from build123d import *

# Parameters (mm, degrees)
PAD_DEPTH     = 20.07
POCKET_DEPTH  = 18.42
SKETCH002_R   = 3
HOLE_DEPTH    = 25
SKETCH003_R   = 3
HOLE001_DEPTH = 25
SKETCH004_R   = 3
HOLE002_DEPTH = 25
SKETCH005_R   = 3
HOLE003_DEPTH = 25
SKETCH006_R   = 3
HOLE004_DEPTH = 25
SKETCH007_R   = 3
HOLE005_DEPTH = 25
SKETCH008_R   = 3
HOLE006_DEPTH = 25
FILLET_R      = 1.5
SKETCH009_R   = 3
HOLE007_DEPTH = 25
SKETCH010_R   = 3
HOLE008_DEPTH = 25
SKETCH011_R   = 3
HOLE009_DEPTH = 25
SKETCH012_R   = 3
HOLE010_DEPTH = 25
SKETCH013_R   = 3
HOLE011_DEPTH = 25
SKETCH014_R   = 3
HOLE012_DEPTH = 25
SKETCH015_R   = 3
HOLE013_DEPTH = 25


with BuildPart() as part:
    # Sketch → Pad (new body)
    with BuildSketch(Plane.XY):
        with BuildLine():
            Line((18.834122, 40.018788), (92.644122, 40.018788))
            ThreePointArc((95.644122, 37.018788), (94.765442, 39.140108), (92.644122, 40.018788))
            Line((95.644122, 37.018788), (95.644122, 5.428788))
            ThreePointArc((92.644122, 2.428788), (94.765442, 3.307467), (95.644122, 5.428788))
            Line((92.644122, 2.428788), (18.834122, 2.428788))
            ThreePointArc((15.834122, 5.428788), (16.712801, 3.307467), (18.834122, 2.428788))
            Line((15.834122, 5.428788), (15.834122, 37.018788))
            ThreePointArc((18.834122, 40.018788), (16.712801, 39.140108), (15.834122, 37.018788))
        make_face()
    extrude(amount=PAD_DEPTH)

    # Sketch001 (on Face9 of Pad) → Pocket (cut)
    with BuildSketch(Plane(origin=(0, 0, 0), x_dir=(1, 0, 0), z_dir=(0, 0, -1))):
        with BuildLine():
            Line((19.344122, -2.933788), (92.134122, -2.933788))
            ThreePointArc((95.134122, -5.933788), (94.255442, -3.812467), (92.134122, -2.933788))
            Line((95.134122, -5.933788), (95.134122, -36.513788))
            ThreePointArc((92.134122, -39.513788), (94.255442, -38.635108), (95.134122, -36.513788))
            Line((92.134122, -39.513788), (19.344122, -39.513788))
            ThreePointArc((16.344122, -36.513788), (17.222801, -38.635108), (19.344122, -39.513788))
            Line((16.344122, -36.513788), (16.344122, -5.933788))
            ThreePointArc((19.344122, -2.933788), (17.222801, -3.812467), (16.344122, -5.933788))
        make_face()
    extrude(amount=-POCKET_DEPTH, mode=Mode.SUBTRACT)

    # Sketch002 (on Face5 of Pocket) → Hole (cut)
    with BuildSketch(Plane.XY.offset(20.07)):
        with Locations((55.739122, 30.621288)):
            Circle(SKETCH002_R)
    extrude(amount=-HOLE_DEPTH, mode=Mode.SUBTRACT)

    # Sketch003 (on Face5 of Hole) → Hole001 (cut)
    with BuildSketch(Plane.XY.offset(20.07)):
        with Locations((45.501322, 30.621288)):
            Circle(SKETCH003_R)
    extrude(amount=-HOLE001_DEPTH, mode=Mode.SUBTRACT)

    # Sketch004 (on Face5 of Hole001) → Hole002 (cut)
    with BuildSketch(Plane.XY.offset(20.07)):
        with Locations((35.290522, 30.621288)):
            Circle(SKETCH004_R)
    extrude(amount=-HOLE002_DEPTH, mode=Mode.SUBTRACT)

    # Sketch005 (on Face5 of Hole002) → Hole003 (cut)
    with BuildSketch(Plane.XY.offset(20.07)):
        with Locations((25.079722, 30.621288)):
            Circle(SKETCH005_R)
    extrude(amount=-HOLE003_DEPTH, mode=Mode.SUBTRACT)

    # Sketch006 (on Face5 of Hole003) → Hole004 (cut)
    with BuildSketch(Plane.XY.offset(20.07)):
        with Locations((65.922922, 30.621288)):
            Circle(SKETCH006_R)
    extrude(amount=-HOLE004_DEPTH, mode=Mode.SUBTRACT)

    # Sketch007 (on Face5 of Hole004) → Hole005 (cut)
    with BuildSketch(Plane.XY.offset(20.07)):
        with Locations((76.133722, 30.621288)):
            Circle(SKETCH007_R)
    extrude(amount=-HOLE005_DEPTH, mode=Mode.SUBTRACT)

    # Sketch008 (on Face5 of Hole005) → Hole006 (cut)
    with BuildSketch(Plane.XY.offset(20.07)):
        with Locations((86.344522, 30.621288)):
            Circle(SKETCH008_R)
    extrude(amount=-HOLE006_DEPTH, mode=Mode.SUBTRACT)

    # Fillet
    fillet_edges = [part.edges().sort_by_distance(p)[0] for p in [
        (55.739122, 40.018788, 20.07),
    ]]
    fillet(fillet_edges, radius=FILLET_R)

    # Sketch009 (on Face8 of Fillet) → Hole007 (cut)
    with BuildSketch(Plane.XY.offset(20.07)):
        with Locations((55.739122, 11.826288)):
            Circle(SKETCH009_R)
    extrude(amount=-HOLE007_DEPTH, mode=Mode.SUBTRACT)

    # Sketch010 (on Face8 of Hole007) → Hole008 (cut)
    with BuildSketch(Plane.XY.offset(20.07)):
        with Locations((45.501322, 11.826288)):
            Circle(SKETCH010_R)
    extrude(amount=-HOLE008_DEPTH, mode=Mode.SUBTRACT)

    # Sketch011 (on Face8 of Hole008) → Hole009 (cut)
    with BuildSketch(Plane.XY.offset(20.07)):
        with Locations((35.290522, 11.826288)):
            Circle(SKETCH011_R)
    extrude(amount=-HOLE009_DEPTH, mode=Mode.SUBTRACT)

    # Sketch012 (on Face8 of Hole009) → Hole010 (cut)
    with BuildSketch(Plane.XY.offset(20.07)):
        with Locations((25.079722, 11.826288)):
            Circle(SKETCH012_R)
    extrude(amount=-HOLE010_DEPTH, mode=Mode.SUBTRACT)

    # Sketch013 (on Face8 of Hole010) → Hole011 (cut)
    with BuildSketch(Plane.XY.offset(20.07)):
        with Locations((65.922922, 11.826288)):
            Circle(SKETCH013_R)
    extrude(amount=-HOLE011_DEPTH, mode=Mode.SUBTRACT)

    # Sketch014 (on Face8 of Hole011) → Hole012 (cut)
    with BuildSketch(Plane.XY.offset(20.07)):
        with Locations((76.133722, 11.826288)):
            Circle(SKETCH014_R)
    extrude(amount=-HOLE012_DEPTH, mode=Mode.SUBTRACT)

    # Sketch015 (on Face8 of Hole012) → Hole013 (cut)
    with BuildSketch(Plane.XY.offset(20.07)):
        with Locations((86.344522, 11.826288)):
            Circle(SKETCH015_R)
    extrude(amount=-HOLE013_DEPTH, mode=Mode.SUBTRACT)


solid = part.part
Here's how the part is built. I have some questions about the finished solid (model axes, mm). A direction names the side the tool comes from. Give positions to 0.01 mm unless a question says otherwise; leave off trailing zeros. Order: outer loops, then holes, each group sorted by start corner. A loop starts at its lowest first (then second) coordinate and runs counter-clockwise, first axis right, second up. Notation, with made-up numbers: M -27.75,52.5 L 19.25,52.5 A25 cw 19.25,66.5 Z; hole C 32,-23.5 d1. An arc over 180 degrees is marked long. Answer as a JSON object with one key per item and string values. Group by question number.
1) We'd pull the mould along Y, two halves only. Please class faces 3 (the cylindrical face through (43.29, 32.65, 19.26)), 4 (the cylindrical face through (16.69, 3.33, 9.16)), 5 (the cylindrical face through (94.789, 39.117, 9.155)): pulls with the +Y half, pulls with the -Y half, needs draft (parallel to the pull), parting line crosses it, or undercut.
2) Suppose I cut it at C-C, the plane x = 52. Write out the boundary of the cut face in (y, z).
3) Suppose I cut it at A-A, the plane z = 12.5. Write out the boundary of the cut face in (x, y).
4) I'm going to push flat-ended pins straight in: pin 1 Ø5 at (x, y) = (35.29, 11.83) entering from -Z; pin 2 Ø7 at (x, y) = (25.08, 30.62) entering from -Z. Where does each tip first touch, or does it pass through?
5) Suppose I cut it at B-B, the plane y = 19.5. Write out the boundary of the cut face in (x, z).
6) Please list where these lines run through material, in increasing order: L1, parallel to Y at x = 89.5, z = 16.25; L2, parallel to X at y = 10, z = 5; L3, parallel to Z at x = 53, y = 16. Write a range as [from, to].
7) Suppose I cut it at D-D, the plane x = 78. Write out the boundary of the cut face in (y, z).
8) On a 3-axis mill with a long thin cutter (end or side, diameter ignored), from which of +Z, -Z, +X, -X, +Y, -Y can I reach the whole of each face in a straight line? I mean faces 1 (the flat face through (55, 2.934, 9)), 2 (the flat face through (95.644, 21, 9)). Say none if no direction works.
Results found:
{
 "1": {"face 3": "undercut", "face 4": "pulls with the -Y half", "face 5": "pulls with the +Y half"},
 "2": {"outline": "M 2.43,0 L 2.93,0 L 2.93,18.42 L 39.51,18.42 L 39.51,0 L 40.02,0 L 40.02,18.57 A1.5 ccw 38.52,20.07 L 3.93,20.07 A1.5 ccw 2.43,18.57 Z"},
 "3": {"outline": "M 15.83,5.43 A3 ccw 18.83,2.43 L 92.64,2.43 A3 ccw 95.64,5.43 L 95.64,37.02 A3 ccw 92.64,40.02 L 18.83,40.02 A3 ccw 15.83,37.02 Z; hole M 16.34,5.93 A3 ccw 19.34,2.93 L 92.13,2.93 A3 ccw 95.13,5.93 L 95.13,36.51 A3 ccw 92.13,39.51 L 19.34,39.51 A3 ccw 16.34,36.51 Z"},
 "4": {"pin 1": "through", "pin 2": "z = 18.42"},
 "5": {"outline": "M 15.83,0 L 16.34,0 L 16.34,18.42 L 95.13,18.42 L 95.13,0 L 95.64,0 L 95.64,18.57 A1.5 ccw 94.14,20.07 L 17.33,20.07 A1.5 ccw 15.83,18.57 Z"},
 "6": {"L1": "[2.43, 2.93], [39.51, 40.02]", "L2": "[15.83, 16.34], [95.13, 95.64]", "L3": "[18.42, 20.07]"},
 "7": {"outline": "M 2.43,0 L 2.93,0 L 2.93,18.42 L 9.48,18.42 L 9.48,20.07 L 3.93,20.07 A1.5 ccw 2.43,18.57 Z; M 14.18,18.42 L 28.27,18.42 L 28.27,20.07 L 14.18,20.07 Z; M 32.97,18.42 L 39.51,18.42 L 39.51,0 L 40.02,0 L 40.02,18.57 A1.5 ccw 38.52,20.07 L 32.97,20.07 Z"},
 "8": {"face 1": "-Z", "face 2": "+Z, -Z, +X, +Y, -Y"}
}
